Design review of the part built by this model. Coordinates are the model's own, in mm. Coordinates: 2 decimals unless noted, no trailing zeros. Write each loop counter-clockwise with the first axis right and the second up, starting at its lowest first coordinate (ties: lowest second). Pieces come first, ordered by that corner, then holes. Notation, with made-up numbers: (70, -8.75) - (110, -8.75) arc R17 cw to (110, 4.25) - close; hole circle Ø5 at (0, 34). An arc over 180 degrees is marked (long way). Use a Markdown table: item, result.
from build123d import *

# Parameters (mm, degrees)
SKETCH1_W           = 14
SKETCH1_H           = 14
BOSS_EXTRUDE2_DEPTH = 65.1
SKETCH2_R           = 2
CUT_EXTRUDE1_DEPTH  = 66.848386465
FILLET1_R           = 7


with BuildPart() as part:
    # Sketch1 → Boss-Extrude2 (new body)
    with BuildSketch(Plane(origin=(0, 0, 0), x_dir=(1, 0, 0), z_dir=(0, 1, 0))):
        Rectangle(SKETCH1_W, SKETCH1_H)
    extrude(amount=BOSS_EXTRUDE2_DEPTH)

    # Sketch2 → Cut-Extrude1 (cut, through all)
    with BuildSketch(Plane(origin=(0, 65.1, 0), x_dir=(1, 0, 0), z_dir=(0, 1, 0))):
        with Locations(Location((0, 0, 0), (0, 0, 270))):
            Circle(SKETCH2_R)
    extrude(amount=-CUT_EXTRUDE1_DEPTH, mode=Mode.SUBTRACT)

    # Fillet1
    fillet1_edges = [part.edges().sort_by_distance(p)[0] for p in [
        (-7, 32.55, 7),
        (-7, 32.55, -7),
        (7, 32.55, -7),
        (7, 32.55, 7),
    ]]
    fillet(fillet1_edges, radius=FILLET1_R - 0.0001)  # a hair under: the kernel refuses the full size


solid = part.part
(1) For L1, parallel to X at y = 14, z = 0; L2, parallel to Z at x = -0.25, y = 62; L3, parallel to X at y = 7.5, z = -1.5, list the stretches that pass through material, from the lowest coordinate up. Write a range as from..to.
Determined:
| item | result |
|---|---|
| L1 | -7..-2, 2..7 |
| L2 | -7..-1.98, 1.98..7 |
| L3 | -6.84..-1.32, 1.32..6.84 |
(2) Draft analysis for pull direction X (two halves, no side actions). For faces 1 (the cylindrical face through (-5, 33, -4.9)), 2 (the cylindrical face through (-2, 33, 0)), 3 (the cylindrical face through (4.9, 33, 5)), state which applies: +X half, -X half, draft (parallel to the pull), parting line (faces both ways), or undercut.
Determined:
| item | result |
|---|---|
| face 1 | -X half |
| face 2 | undercut |
| face 3 | +X half |
(3) Take a section at B-B on z = -1.25. Write out the cut boundary in (x, y), and give its area (3 significant figures).
Determined:
| item | result |
|---|---|
| outline | (-6.89, 0) - (-1.56, 0) - (-1.56, 65.1) - (-6.89, 65.1) - close; (1.56, 0) - (6.89, 0) - (6.89, 65.1) - (1.56, 65.1) - close |
| area | 693 mm2 |
(4) For pin 1 (5 mm diameter, centred on y = 19, z = -5.5, fed in from -X); pin 2 (2 mm diameter, centred on x = 5, y = 32.5, fed in from +Z), all flat-tipped, find the tip position at first contact; note any pin that passes through.
Determined:
| item | result |
|---|---|
| pin 1 | x = -6.32 |
| pin 2 | z = 5.74 |
(5) Take a section at C-C on x = 3.25. Write out the cut boundary in (y, z), and give its area (3 significant figures).
Determined:
| item | result |
|---|---|
| outline | (0, -6.2) - (65.1, -6.2) - (65.1, 6.2) - (0, 6.2) - close |
| area | 807 mm2 |
(6) Take a section at D-D on z = 3.5. Write out the cut boundary in (x, y), and give its area (3 significant figures).
Determined:
| item | result |
|---|---|
| outline | (-6.06, 0) - (6.06, 0) - (6.06, 65.1) - (-6.06, 65.1) - close |
| area | 789 mm2 |
